from build123d import *

# Parameters (mm, degrees)
BOSS_EXTRUDE1_DEPTH = 40
CHAMFER1_SIZE       = 20
CUT_EXTRUDE1_DEPTH  = 20
SKETCH3_W           = 10
SKETCH3_H           = 15
CUT_EXTRUDE2_DEPTH  = 70


with BuildPart() as part:
    # Sketch1 → Boss-Extrude1 (new body)
    with BuildSketch(Plane(origin=(0, 0, 0), x_dir=(1, 0, 0), z_dir=(0, 1, 0))):
        Polygon((0, 0), (30, 0), (30, 10), (60, 10), (60, -60), (40, -60), (40, -70), (30, -70), (30, -60), (10, -60), (10, -70), (0, -70), align=None)
    extrude(amount=BOSS_EXTRUDE1_DEPTH)

    # Chamfer1
    chamfer1_edges = [part.edges().sort_by_distance(p)[0] for p in [
        (5, 40, 70),
    ]]
    chamfer(chamfer1_edges, length=CHAMFER1_SIZE)

    # Sketch2 → Cut-Extrude1 (cut)
    with BuildSketch(Plane(origin=(60, 0, 0), x_dir=(0, 0, -1), z_dir=(1, 0, 0))):
        Polygon((0, 30), (0, 40), (-50, 40), (-60, 30), (-60, 0), (-50, 0), (-20, 30), align=None)
    extrude(amount=-CUT_EXTRUDE1_DEPTH, mode=Mode.SUBTRACT)

    # Sketch3 → Cut-Extrude2 (cut)
    with BuildSketch(Plane.XY.offset(70)):
        with Locations((55, 22.5)):
            Rectangle(SKETCH3_W, SKETCH3_H)
    extrude(amount=-CUT_EXTRUDE2_DEPTH, mode=Mode.SUBTRACT)


solid = part.part
CAD build for the part. Positions are in the model's coordinates, mm. A direction names the side the tool comes from. Round coordinates to 2 decimals unless told otherwise and drop trailing zeros. Write each loop counter-clockwise with the first axis right and the second up, starting at its lowest first coordinate (ties: lowest second). Pieces come first, ordered by that corner, then holes.
(1) Mould opens along X. For faces 6 (the face through (55, 15, 18)), 7 (the face through (30, 20, -5)), 8 (the face through (10, 11, 65)) say: pulls with the +X half, pulls with the -X half, needs draft (parallel to the pull), parting line crosses it, or undercut.
(2) Slice it at B-B, the plane y = 33. Write the cut outline in (x, z), and give its area (3 significant figures).
(3) Slice it at A-A, the plane z = 61.5. Write the cut outline in (x, y).
(4) Drop flat-ended pins along their axis: P1, Ø5, axis at x = 56.5, z = 9, coming from the +Y side; P2, Ø7.5, axis at y = 23.5, z = 12.5, coming from the +X side; P3, Ø1, axis at x = 33, y = 36, coming from the +Z side; P4, Ø3, axis at y = 9.5, z = 66, coming from the -X side. Give the stop position or say it passes through.
(5) Slice it at D-D, the plane x = 44.5. Write the cut outline in (y, z), and give its area (3 significant figures).
(6) 3-axis set-ups, long thin cutter, end or side, ignore diameter. For faces 1 (the face through (50, 22, 14)), 2 (the face through (24, 40, 20)), 3 (the face through (45, 20, -10)), 4 (the face through (30, 11, 65)), 5 (the face through (15, 20, 0)): which of +Z, -Z, +X, -X, +Y, -Y reach the whole face in a straight line?
(7) Probe line 1 along Z through (x, y) = (12, 27.5); line 2 along X through (y, z) = (34, 26); line 3 along Y through (x, z) = (44.5, 10). List the from-to ranges inside material, lowest first.
(8) Slice it at C-C, the plane z = 22.5. Write the cut outline in (x, y).
From the geometry:
1. face 6: needs draft
1. face 7: pulls with the -X half
1. face 8: undercut
2. outline: (0, 0) - (30, 0) - (30, -10) - (60, -10) - (60, 0) - (40, 0) - (40, 57) - (0, 57) - close
2. area: 2,580 mm2
3. outline: (0, 0) - (10, 0) - (10, 28.5) - (0, 28.5) - close; (30, 0) - (40, 0) - (40, 28.5) - (30, 28.5) - close
4. P1: stops at y = 15
4. P2: stops at x = 50
4. P3: stops at z = 54.5
4. P4: stops at x = 0
5. outline: (0, -10) - (40, -10) - (40, 0) - (30, 0) - (30, 20) - (0, 50) - close
5. area: 1,450 mm2
6. face 1: +Z, +X, +Y
6. face 2: +Z, -Z, +X, -X, +Y
6. face 3: -Z, +X, -X, +Y, -Y
6. face 4: +Z, +Y, -Y
6. face 5: -Z, -X, +Y, -Y
7. line 1: z = 0 to 60
7. line 2: x = 0 to 40
7. line 3: y = 0 to 30
8. outline: (0, 0) - (60, 0) - (60, 15) - (50, 15) - (50, 27.5) - (40, 27.5) - (40, 40) - (0, 40) - close
